Autodesk Inventor part; units mm, degrees
ref_plane "Płaszczyzna konstrukcyjna1" through (0, 2, 0) normal (0, -1, 0) x (1, 0, 0)
ref_plane "YZ Plane" through (0, 0, 0) normal (1, 0, 0) x (0, 1, 0)
ref_plane "XZ Plane" through (0, 0, 0) normal (0, 1, 0) x (-1, 0, 0)
sketch "Szkic1" plane through (0, 0, 0) normal (0, 1, 0) x (-1, 0, 0)
  circle A0 centre (0, 0) radius 6
  dimension "d0" = 12
extrude "Wyciągnięcie proste1" add sketch "Szkic1" along normal blind 53
sketch "Szkic2" plane through (0, 53, 0) normal (0, 1, 0) x (1, 0, 0)
  point P0 (0, 0)
  point P1 (0, 0)
ref_plane "Płaszczyzna konstrukcyjna1" through (0, 2, 0) normal (0, -1, 0) x (1, 0, 0)
hole "Otwór1" at (0, 53, 0) direction (0, -1, 0) diameter 11 depth 51
sketch "Szkic3" plane through (0, 0, 0) normal (0, -1, 0) x (1, 0, 0)
  point P0 (0, 0)
  point P1 (0, 0)
hole "Otwór2" at (0, 0, 0) direction (0, 1, 0) diameter 7 end through all
fillet "Zaokrąglenie1" radius 1 1 edges at (6, 0, 0)
properties part number "Jack_obudowa"
Read the model definition and answer for the solid it produces. Units are mm, in the model's axes. A direction names the side the tool comes from. Round coordinates to 2 decimals unless told otherwise and drop trailing zeros. Order: outer loops, then holes, each group sorted by start corner. A loop starts at its lowest first (then second) coordinate and runs counter-clockwise, first axis right, second up. Notation, with made-up numbers: (15, -9.5) - (74, -9.5) arc R21 ccw to (74, 26.5) - close; hole circle Ø1 at (81, 52). An arc over 180 degrees is marked (long way). Use one line per item in the form item = value. Start each with the question number.
(1) Flat-ended cylindrical pins translate along their axes: pin 1 Ø1.5 at (y, z) = (44.5, 3.5) entering from -X; pin 2 Ø3.5 at (x, z) = (1, 2) entering from +Y; pin 3 Ø6.5 at (x, z) = (0, 0) entering from -Y; pin 4 Ø2 at (x, y) = (-1.5, 36) entering from +Z. Find the tip coordinate at first contact, or state that the pin passes through.
(2) Determine the mould class of faces 3 (the face through (6, 27, 0)), 4 (the face through (-3, 53, -5)), 5 (the face through (1.341, 1.014, -3.233)) for opening direction X: +X half, -X half, draft (parallel to the pull), parting line (faces both ways), or undercut.
(3) Find the intervals of material crossed by line 1 along Z through (x, y) = (0, 14); line 2 along Z through (x, y) = (0, 1.3); line 3 along X through (y, z) = (23.5, -3.75), in increasing order. Write a range as from..to.
(4) The part is cut by section B-B (x = 0). Give the vertices of the cut face in (y, z).
(5) For faces 1 (the face through (0, 2, 4)), 2 (the face through (-2.2, 0, -3.3)), determine the directions among +Z, -Z, +X, -X, +Y, -Y from which every point of the face is accessible in a straight line to the end or side of a thin tool.
(6) The part is cut by section A-A (z = 0). Give the vertices of the cut face in (x, y), then the cut area to 3 significant figures.
(7) The part is cut by section C-C (y = 16). Give the vertices of the cut face in (x, z).
Checked values:
q1.pin_1 = -5.33
q1.pin_2 = 2
q1.pin_3 = through
q1.pin_4 = 5.98
q2.face_3 = parting line
q2.face_4 = draft
q2.face_5 = undercut
q3.line_1 = -6..-5.5, 5.5..6
q3.line_2 = -6..-3.5, 3.5..6
q3.line_3 = -4.68..-4.02, 4.02..4.68
q4.outline = (0, -5) arc R1 ccw to (1, -6) - (53, -6) - (53, -5.5) - (2, -5.5) - (2, -3.5) - (0, -3.5) - close; (0, 3.5) - (2, 3.5) - (2, 5.5) - (53, 5.5) - (53, 6) - (1, 6) arc R1 ccw to (0, 5) - close
q5.face_1 = +Y
q5.face_2 = +Z, -Z, +X, -X, -Y
q6.outline = (-6, 1) arc R1 ccw to (-5, 0) - (-3.5, 0) - (-3.5, 2) - (-5.5, 2) - (-5.5, 53) - (-6, 53) - close; (3.5, 0) - (5, 0) arc R1 ccw to (6, 1) - (6, 53) - (5.5, 53) - (5.5, 2) - (3.5, 2) - close
q6.area = 60.6 mm^2
q7.outline = circle Ø12 at (0, 0); hole circle Ø11 at (0, 0)
